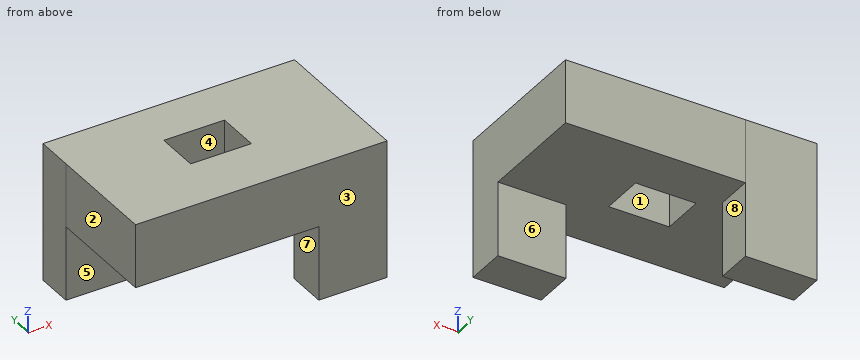
```python
from build123d import *

# Parameters (mm, degrees)
F0_W     = 24.078095
F0_H     = 12.475135
F0_W_2   = 22.912228
F0_H_2   = 13.509782
F0_W_3   = 20.404858
F0_H_3   = 14.665992
F1_DEPTH = 46.4
F2_DEPTH = 25


with BuildPart() as f1:
    # F0 (on Top) → F1 (new body)
    with BuildSketch(Plane.XY):
        with Locations((-28.458583, 17.7153)):
            Rectangle(F0_W, F0_H)
        with Locations((32.498623, -19.66734)):
            Rectangle(F0_W_2, F0_H_2)
        Polygon((43.954737, 23.952868), (-16.419536, 23.952868), (-16.419536, 11.477733), (-40.497631, 11.477733), (-40.497631, -26.422231), (21.042509, -26.422231), (21.042509, -12.912449), (43.954737, -12.912449), align=None)
        Rectangle(F0_W_3, F0_H_3, mode=Mode.SUBTRACT)
    extrude(amount=F1_DEPTH)

    # F0 (on Top) → F2 (cut)
    with BuildSketch(Plane.XY):
        Polygon((43.954737, 23.952868), (-16.419536, 23.952868), (-16.419536, 11.477733), (-40.497631, 11.477733), (-40.497631, -26.422231), (21.042509, -26.422231), (21.042509, -12.912449), (43.954737, -12.912449), align=None)
        Rectangle(F0_W_3, F0_H_3, mode=Mode.SUBTRACT)
    extrude(amount=F2_DEPTH, mode=Mode.SUBTRACT)


solid = f1.part
```
For this review, take the finished solid that the model builds, in its own axes (mm). Face numbers are marked on the shaded views. A direction names the side the tool comes from. Coordinates: 2 decimals unless noted, no trailing zeros. Order: outer loops, then holes, each group sorted by start corner. A loop starts at its lowest first (then second) coordinate and runs counter-clockwise, first axis right, second up. Notation, with made-up numbers: (2.25, 69.25) -> (11.25, 69.25) arc R23 ccw to (11.25, 91.25) -> close; hole circle Ø9 at (-39, 13.25). An arc over 180 degrees is marked (long way). Use CSV: the item, a comma, the result in double quotes. Start each with the question number.
Item 1: For the marked faces 4, 5, 6, 7 and 8, list the 3-axis set-ups (+Z, -Z, +X, -X, +Y, -Y) from which the entire face can be reached by the end or side of a thin tool; tool diameter is ignored.
Item 2: Insertion check: pin 1 (18.5 mm diameter, centred on x = 37, z = 6.5, fed in from +Y); pin 2 (12 mm diameter, centred on x = 5, y = 13, fed in from -Z); pin 3 (7 mm diameter, centred on x = -31, z = 14.5, fed in from -Y). Each pin has a flat end and moves straight along its axis. Give the tip position at first contact, or say it passes through.
Item 3: Wall thickness on probe 1 along Y at (x, z) = (9.5, 31); probe 2 along X at (y, z) = (6.5, 30); probe 3 along Z at (x, y) = (37.5, 1): over which ranges is each line inside the solid? List them lowest first.
Item 4: We need section D-D, the plane x = 22. Give the boundary of the cut face in (y, z).
Item 5: We need section C-C, the plane z = 38.5. Give the boundary of the cut face in (x, y), then the cut area to 3 significant figures.
Item 6: We need section B-B, the plane y = -5.5. Give the boundary of the cut face in (x, z).
Item 7: Draft analysis for pull direction Y (two halves, no side actions). For the marked faces 1, 2 and 3, state which applies: pulls with the +Y half, pulls with the -Y half, needs draft (parallel to the pull), parting line crosses it, or undercut.
Item 8: We need section A-A, the plane z = 6.5. Give the boundary of the cut face in (x, y), then the cut area to 3 significant figures.
Derived:
1,face 4,"+Z, -Z"
1,face 5,"-Z, +X, -X, -Y"
1,face 6,"-Z, +X, -X, +Y"
1,face 7,"-Z, -X, +Y, -Y"
1,face 8,"-Z, +X, +Y, -Y"
2,pin 1,"stops at y = -12.91"
2,pin 2,"stops at z = 25"
2,pin 3,"stops at y = 11.48"
3,probe 1,"y = -26.42 to -7.33, 7.33 to 23.95"
3,probe 2,"x = -40.5 to -10.2, 10.2 to 43.95"
3,probe 3,"z = 25 to 46.4"
4,outline,"(-26.42, 0) -> (-12.91, 0) -> (-12.91, 25) -> (23.95, 25) -> (23.95, 46.4) -> (-26.42, 46.4) -> close"
5,outline,"(-40.5, -26.42) -> (43.95, -26.42) -> (43.95, 23.95) -> (-40.5, 23.95) -> close; hole (-10.2, -7.33) -> (10.2, -7.33) -> (10.2, 7.33) -> (-10.2, 7.33) -> close"
5,area,"3,960 mm^2"
6,outline,"(-40.5, 25) -> (-10.2, 25) -> (-10.2, 46.4) -> (-40.5, 46.4) -> close; (10.2, 25) -> (43.95, 25) -> (43.95, 46.4) -> (10.2, 46.4) -> close"
7,face 1,"undercut"
7,face 2,"needs draft"
7,face 3,"pulls with the -Y half"
8,outline,"(-40.5, 11.48) -> (-16.42, 11.48) -> (-16.42, 23.95) -> (-40.5, 23.95) -> close; (21.04, -26.42) -> (43.95, -26.42) -> (43.95, -12.91) -> (21.04, -12.91) -> close"
8,area,"610 mm^2"
